Read the model definition and answer for the solid it produces. Units are mm, in the model's axes. Give positions to 0.01 mm unless a question says otherwise; leave off trailing zeros. Write each loop counter-clockwise with the first axis right and the second up, starting at its lowest first coordinate (ties: lowest second). Pieces come first, ordered by that corner, then holes.
```python
from build123d import *

# Parameters (mm, degrees)
SKETCH1_R           = 18.25625
BOSS_EXTRUDE1_DEPTH = 101.6
CHAMFER1_SIZE       = 25.4
CHAMFER1_SIZE2      = 3.96875
CHAMFER2_SIZE       = 3.96875
CHAMFER2_SIZE2      = 25.4


with BuildPart() as part:
    # Sketch1 → Boss-Extrude1 (new body, symmetric)
    with BuildSketch(Plane.XY):
        Circle(SKETCH1_R)
    extrude(amount=BOSS_EXTRUDE1_DEPTH, both=True)

    # Chamfer1
    chamfer1_edges = [part.edges().sort_by_distance(p)[0] for p in [
        (-18.25625, 0, 101.6),
    ]]
    chamfer1_side = [part.faces().sort_by_distance(p)[0] for p in [
        (-18.25625, 0, 0),
    ]]
    chamfer(chamfer1_edges, length=CHAMFER1_SIZE, length2=CHAMFER1_SIZE2, reference=chamfer1_side[0])

    # Chamfer2
    chamfer2_edges = [part.edges().sort_by_distance(p)[0] for p in [
        (-18.25625, 0, -101.6),
    ]]
    chamfer2_side = [part.faces().sort_by_distance(p)[0] for p in [
        (0, 0, -101.6),
    ]]
    chamfer(chamfer2_edges, length=CHAMFER2_SIZE, length2=CHAMFER2_SIZE2, reference=chamfer2_side[0])


solid = part.part
```
Item 1: Find the intervals of material crossed by line 1 along Y through (x, z) = (-1, -57); line 2 along Y through (x, z) = (12, -15); line 3 along X through (y, z) = (11, 61), in increasing order.
Result set:
line 1: y = -18.23 to 18.23
line 2: y = -13.76 to 13.76
line 3: x = -14.57 to 14.57
Item 2: Section C-C (z = 52) is taken. Write down the section's boundary in (x, y).
Result set:
outline: circle Ø36.51 at (0, 0)
Item 3: Each of these flat-tipped pins is pushed along its axis until it touches: pin 1 Ø8 at (y, z) = (-5.5, -26.5) entering from +X; pin 2 Ø8 at (x, z) = (9, -8) entering from +Y; pin 3 Ø12 at (x, z) = (13.5, -57) entering from -Y. Where does it stop, or does it pass through?
Result set:
pin 1: stops at x = 18.19
pin 2: stops at y = 17.56
pin 3: stops at y = -16.64
Item 4: Section A-A (y = 0) is taken. Write down the section's boundary in (x, z), and give its area (3 significant figures).
Result set:
outline: (-18.26, -76.2) - (-14.29, -101.6) - (14.29, -101.6) - (18.26, -76.2) - (18.26, 76.2) - (14.29, 101.6) - (-14.29, 101.6) - (-18.26, 76.2) - close
area: 7,220 mm2
